Here's how the part is built. I have some questions about the finished solid (model axes, mm). A direction names the side the tool comes from. Round coordinates to 2 decimals unless told otherwise and drop trailing zeros. Loops run counter-clockwise (first coordinate to the right, second up) from the corner with the lowest first, then second, coordinate; pieces in that order, holes last. Notation, with made-up numbers: (59, 6.25) -> (118, 6.25) arc R20 cw to (118, 45.25) -> close; hole circle Ø9 at (50, -9). An arc over 180 degrees is marked (long way). Use one line per item in the form item = value. Start each with the question number.
Item 1: I'm going to push flat-ended pins straight in: pin 1 Ø10 at (x, z) = (-7, 26) entering from +Y; pin 2 Ø8 at (y, z) = (21, 25) entering from -X; pin 3 Ø10 at (x, z) = (-6, 15.5) entering from -Y. Where does each tip first touch, or does it pass through?
Item 2: If I drill on L1, parallel to X at y = -8.5, z = 26.5; L2, parallel to X at y = -6.5, z = 17.5; L3, parallel to X at y = -6.5, z = 8.5, over which ranges is the centre line in solid material (lowest first)? Write a range as [from, to].
Item 3: If we section it at D-D (z = 17.5): Write out the boundary of the cut face in (x, y).
Item 4: Thinking about a two-plate mould opening in Z: for faces 1 (the face through (-1, 39.2, 17)), 2 (the face through (-1, -40, 17)), 3 (the face through (-26, 9, 0.8)), 4 (the face through (-39.2, -1, 17)), which applies, released by +Z, released by -Z, zero draft, split by the parting line, or undercut?
Item 5: If we section it at A-A (z = 6.5): Write out the boundary of the cut face in (x, y).
Item 6: For faces 5 (the face through (-1, 40, 17)), 6 (the face through (5.23, 23.53, 11.83)), 7 (the face through (40, -1, 17)), 8 (the face through (39.2, -1, 17)), which set-ups out of +Z, -Z, +X, -X, +Y, -Y let a thin tool reach every point of the face, with its end or its side?
```python
from build123d import *

# Parameters (mm, degrees)
F0_W             = 80
F0_H             = 80
F1_DEPTH         = 34
F2_T             = -0.8
F3_R             = 25
F4_DEPTH         = 24
F4_TAPER         = 0.5
F5_T1_DEPTH      = 78.4
F5_T3_DEPTH      = 78.4
F6_W             = 80
F6_H             = 80
F6_W_2           = 76
F6_H_2           = 76
F7_DEPTH         = 0.05
F8_SIZE          = 1.19999
F11_DEPTH        = 34.05
F11_COPIES_COUNT = 4


# Not quite as in the source:
# - a fillet or chamfer that OpenCascade refuses, or shapes differently, is made with other operations: its cross-section is extruded or revolved along the edge and cut away or added
# - a fillet or chamfer is up to 0.001 mm smaller than in the source, because OpenCascade refuses the exact size
# - a pattern or mirror of a feature is missing from the dataset's text; its kind, count and spacing are read off the source's solid


with BuildPart() as f1:
    # F0 (on Top) → F1 (new body)
    with BuildSketch(Plane.XY):
        Rectangle(F0_W, F0_H)
    extrude(amount=F1_DEPTH)

    # F2
    f2_openings = [f1.faces().sort_by_distance(p)[0] for p in [
        (0, 0, 34),
    ]]
    offset(amount=F2_T, openings=f2_openings)

    # F3 (on face) → F4 (join)
    with BuildSketch(Plane.XY.offset(0.8)):
        Circle(F3_R)
    extrude(amount=F4_DEPTH, taper=F4_TAPER)

    # F5: chamfer of 1.2 on 5 edges, made by hand

    # F5_s2 → F5_t1 (join)
    with BuildSketch(Plane.XZ.offset(-39.2)):
        Polygon((-39.2, 2), (-38, 0.8), (-39.2, 0.8), align=None)
        Polygon((39.2, 2), (38, 0.8), (39.2, 0.8), align=None)
    extrude(amount=F5_T1_DEPTH)

    # F5_s4 → F5_t3 (join)
    with BuildSketch(Plane.YZ.offset(-39.2)):
        Polygon((-39.2, 2), (-38, 0.8), (-39.2, 0.8), align=None)
        Polygon((39.2, 2), (38, 0.8), (39.2, 0.8), align=None)
    extrude(amount=F5_T3_DEPTH)

    # F5_s5 → F5_t6 (revolve)
    with BuildSketch(Plane.XZ):
        Polygon((26.1895734527, 0.8), (24.989619145, 1.9895281574), (25, 0.8), align=None)
    revolve(axis=Axis((0, 0, 0.8), (0, 0, -1)))

    # F6 (on face) → F7 (join)
    with BuildSketch(Plane.XY.offset(34)):
        Rectangle(F6_W, F6_H)
        Rectangle(F6_W_2, F6_H_2, mode=Mode.SUBTRACT)
    extrude(amount=F7_DEPTH)

    # F8 (size 1.2 in the source; OpenCascade refuses exactly that, so slightly less here)
    f8_edges = [f1.edges().sort_by_distance(p)[0] for p in [
        (0, -39.2, 34),
        (-39.2, 0, 34),
        (-39.2, -39.2, 18),
        (-39.2, 39.2, 18),
        (0, 39.2, 34),
        (39.2, 0, 34),
        (39.2, 39.2, 18),
        (39.2, -39.2, 18),
    ]]
    chamfer(f8_edges, length=F8_SIZE)

    # F9: chamfer of 0.8 on 1 edges, made by hand

    # F9_s1 → F9_t2 (revolve, cut)
    with BuildSketch(Plane.XZ):
        Polygon((24.7975364014, 24.0000304615), (23.990555173, 24.8), (24.790555173, 24.8), align=None)
    revolve(axis=Axis((0, 0, 24.8), (0, 0, -1)), mode=Mode.SUBTRACT)

    # F10 (on face) → F11 (join, through all)
    with BuildSketch(Plane(origin=(0, 0, 0), x_dir=(1, 0, 0), z_dir=(0, 0, -1))):
        with BuildLine():
            Line((-39.1612012219, 39.7268866468), (-39.7171572875, 40.2828427125))
            ThreePointArc((-39.7171572875, 40.2828427125), (-39.7171572875, 39.7171572875), (-40.2828427125, 39.7171572875))
            Line((-40.2828427125, 39.7171572875), (-39.7268866468, 39.1612012219))
            Line((-39.7268866468, 39.1612012219), (-39.1612012219, 39.7268866468))
        make_face()
        with BuildLine():
            ThreePointArc((-40.2828427125, 39.7171572875), (-39.7171572875, 39.7171572875), (-39.7171572875, 40.2828427125))
            Line((-39.7171572875, 40.2828427125), (-42.5455844123, 43.1112698372))
            ThreePointArc((-42.5455844123, 43.1112698372), (-43.1112698372, 43.1112698372), (-43.1112698372, 42.5455844123))
            Line((-43.1112698372, 42.5455844123), (-40.2828427125, 39.7171572875))
        make_face()
    f11 = extrude(amount=-F11_DEPTH)

    # F11_copies: F11 ×4 about axis
    f11_copies_axis = Axis((0, 0, 0), (0, 0, 1))
    for i in range(1, F11_COPIES_COUNT):
        add(f11.rotate(f11_copies_axis, i * 360 / F11_COPIES_COUNT))

    # F12 (on Front) → F13 (revolve, cut)
    with BuildSketch(Plane.XZ):
        Polygon((-23.9975059387, 24.0000304615), (-24.2264749318, -2.2372173829), (0, -2.2372173829), (0, 24.0000304615), align=None)
    revolve(axis=Axis((0, 0, 10.8814065393), (0, 0, 1)), mode=Mode.SUBTRACT)


solid = f1.part
```
Values found:
q1.pin_1 = 40
q1.pin_2 = -40
q1.pin_3 = -40
q2.L1 = [-40, -39.2], [39.2, 40]
q2.L2 = [-40, -39.2], [-23.99, -23.16], [23.16, 23.99], [39.2, 40]
q2.L3 = [-40, -39.2], [-24.07, -23.24], [23.24, 24.07], [39.2, 40]
q3.outline = (-43.11, -42.55) arc R0.4 ccw to (-42.55, -43.11) -> (-39.43, -40) -> (39.43, -40) -> (42.55, -43.11) arc R0.4 ccw to (43.11, -42.55) -> (40, -39.43) -> (40, 39.43) -> (43.11, 42.55) arc R0.4 ccw to (42.55, 43.11) -> (39.43, 40) -> (-39.43, 40) -> (-42.55, 43.11) arc R0.4 ccw to (-43.11, 42.55) -> (-40, 39.43) -> (-40, -39.43) -> close; circle Ø49.71 at (0, 0); hole (-39.2, -38) -> (-38, -39.2) -> (38, -39.2) -> (39.2, -38) -> (39.2, 38) -> (38, 39.2) -> (-38, 39.2) -> (-39.2, 38) -> close; hole circle Ø48.11 at (0, 0)
q4.face_1 = undercut
q4.face_2 = zero draft
q4.face_3 = released by +Z
q4.face_4 = undercut
q5.outline = (-43.11, -42.55) arc R0.4 ccw to (-42.55, -43.11) -> (-39.43, -40) -> (39.43, -40) -> (42.55, -43.11) arc R0.4 ccw to (43.11, -42.55) -> (40, -39.43) -> (40, 39.43) -> (43.11, 42.55) arc R0.4 ccw to (42.55, 43.11) -> (39.43, 40) -> (-39.43, 40) -> (-42.55, 43.11) arc R0.4 ccw to (-43.11, 42.55) -> (-40, 39.43) -> (-40, -39.43) -> close; circle Ø49.9 at (0, 0); hole (-39.2, -38) -> (-38, -39.2) -> (38, -39.2) -> (39.2, -38) -> (39.2, 38) -> (38, 39.2) -> (-38, 39.2) -> (-39.2, 38) -> close; hole circle Ø48.3 at (0, 0)
q6.face_5 = +Z, -Z, +Y
q6.face_6 = -Z
q6.face_7 = +Z, -Z, +X
q6.face_8 = none
